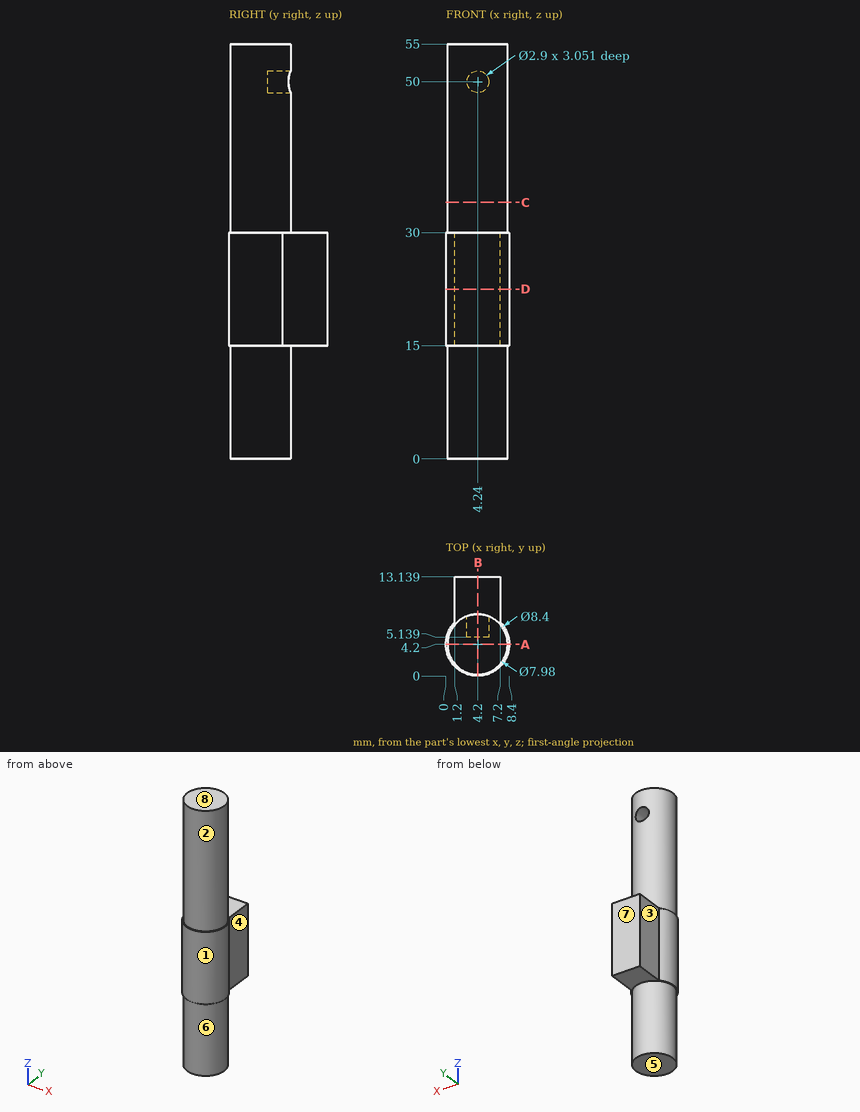
Source: three-view drawing plus pictorial views. Frame: mm from the lowest corner of the part. A direction names the side the tool comes from. Round coordinates to 2 decimals unless told otherwise and drop trailing zeros. Order: outer loops, then holes, each group sorted by start corner. A loop starts at its lowest first (then second) coordinate and runs counter-clockwise, first axis right, second up. Notation, with made-up numbers: (36, -1) -> (41, -1) arc R25 ccw to (41, 21) -> close; hole circle Ø10 at (54.5, 34.5). An arc over 180 degrees is marked (long way). Use CSV: the item, a comma, the result in double quotes. Start each with the question number.
1) Material intervals for line 1 along Z through (x, y) = (4.24, 6.1); line 2 along Z through (x, y) = (6.5, 7.75); line 3 along X through (y, z) = (6.55, 50) (1 decimal), sorted ascending. Write a range as from..to.
2) Section C-C (z = 34). Return the cut outline in (x, y).
3) Section B-B (x = 4.24). Return the cut outline in (y, z).
4) First-contact query: pin 1 Ø4 at (x, z) = (1.5, 38.5) entering from +Y; pin 2 Ø1.8 at (y, z) = (10.5, 24.5) entering from +X; pin 3 Ø0.9 at (x, z) = (4, 50) entering from +Y. Flat tips, straight axial feed; report the tip coordinate or a pass-through.
5) Section D-D (z = 22.5). Return the cut outline in (x, y).
6) Section A-A (y = 4.2). Return the cut outline in (x, z).
7) Draft query along Y for the marked faces 6, 7 and 8. Return one class per face: +Y half, -Y half, draft (parallel to the pull), parting line (faces both ways), or undercut.
8) Set-up query: the marked faces 1, 2, 3, 4 and 5. Return all of +Z, -Z, +X, -X, +Y, -Y with unobstructed straight access to the full face (end or side cutting, diameter ignored); none if empty.
Returned:
1,line 1,"z = 0..48.55, 51.45..55"
1,line 2,"z = 15..30"
1,line 3,"x = 1..2.8, 5.7..7.4"
2,outline,"circle Ø7.98 at (4.2, 4.2)"
3,outline,"(0, 15) -> (0.21, 15) -> (0.21, 0) -> (8.19, 0) -> (8.19, 15) -> (13.14, 15) -> (13.14, 30) -> (8.19, 30) -> (8.19, 48.55) -> (5.14, 48.55) -> (5.14, 51.45) -> (8.19, 51.45) -> (8.19, 55) -> (0.21, 55) -> (0.21, 30) -> (0, 30) -> close"
4,pin 1,"stops at y = 8.13"
4,pin 2,"stops at x = 7.2"
4,pin 3,"stops at y = 5.14"
5,outline,"(1.2, 7.14) arc R4.2 ccw (long way) to (7.2, 7.14) -> (7.2, 13.14) -> (1.2, 13.14) -> close"
6,outline,"(0, 15) -> (0.21, 15) -> (0.21, 0) -> (8.19, 0) -> (8.19, 15) -> (8.4, 15) -> (8.4, 30) -> (8.19, 30) -> (8.19, 55) -> (0.21, 55) -> (0.21, 30) -> (0, 30) -> close"
7,face 6,"parting line"
7,face 7,"+Y half"
7,face 8,"draft"
8,face 1,"+Z, -Z"
8,face 2,"+Z"
8,face 3,"+Z, -Z, -X, +Y"
8,face 4,"+Z, -Z, +X, +Y"
8,face 5,"-Z, +X, -X, +Y, -Y"
